The figure shows three views and two pictorial views of one solid part (mm, origin at its lowest corner). Answer the questions. A direction names the side the tool comes from. Round coordinates to 2 decimals unless told otherwise and drop trailing zeros. Write each loop counter-clockwise with the first axis right and the second up, starting at its lowest first coordinate (ties: lowest second). Pieces come first, ordered by that corner, then holes.
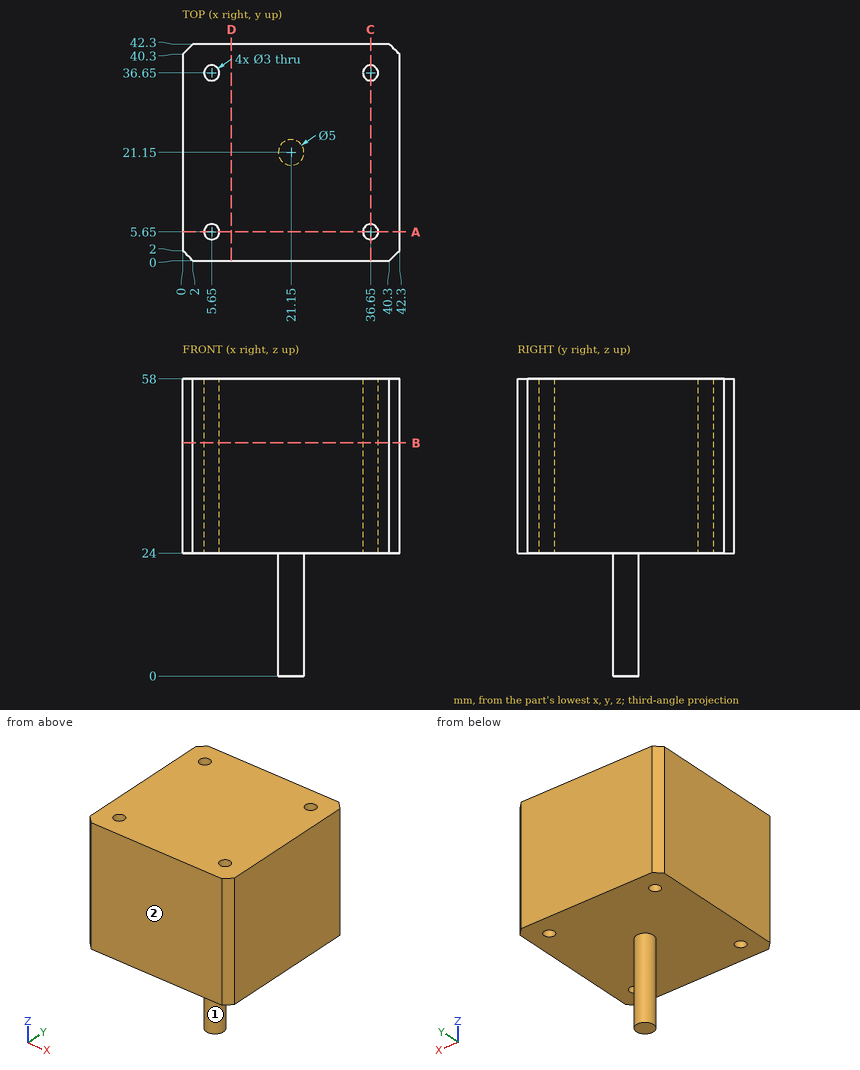
Q1. Section D-D (x = 9.5) is taken. Determine the outline of the cut face in (y, z), then the cut area to 3 significant figures.
Verdict:
outline: (0, 24) - (42.3, 24) - (42.3, 58) - (0, 58) - close
area: 1,440 mm2
Q2. Which of the six approach directions +Z, -Z, +X, -X, +Y, -Y give full straight-line access (tool end or side, diameter ignored) to the marked faces 1 and 2?
Verdict:
face 1: -Z
face 2: +Z, -Z, +X, -X, -Y
Q3. Section A-A (y = 5.65) is taken. Determine the outline of the cut face in (x, z), then the cut area to 3 significant figures.
Verdict:
outline: (0, 24) - (4.15, 24) - (4.15, 58) - (0, 58) - close; (7.15, 24) - (35.15, 24) - (35.15, 58) - (7.15, 58) - close; (38.15, 24) - (42.3, 24) - (42.3, 58) - (38.15, 58) - close
area: 1,230 mm2
Q4. Section B-B (z = 45.5) is taken. Determine the outline of the cut face in (x, y), then the cut area to 3 significant figures.
Verdict:
outline: (0, 2) - (2, 0) - (40.3, 0) - (42.3, 2) - (42.3, 40.3) - (40.3, 42.3) - (2, 42.3) - (0, 40.3) - close; hole circle Ø3 at (5.65, 5.65); hole circle Ø3 at (5.65, 36.65); hole circle Ø3 at (36.65, 5.65); hole circle Ø3 at (36.65, 36.65)
area: 1,750 mm2
Q5. A flat-ended cylindrical pin translates along its axis: pin 1 Ø1 at (x, y) = (36.5, 13) entering from -Z. Find the tip coordinate at first contact, or state that the pin passes through.
Verdict:
pin 1: stops at z = 24
Q6. Straight lines are drawn through the part: probe 1 along Y at (x, z) = (36.65, 41); probe 2 along Y at (x, z) = (5, 45); probe 3 along Z at (x, y) = (6, 4). For each, find the intervals that lie inside material, in ascending order.
Verdict:
probe 1: y = 0 to 4.15, 7.15 to 35.15, 38.15 to 42.3
probe 2: y = 0 to 4.3, 7 to 35.3, 38 to 42.3
probe 3: z = 24 to 58
